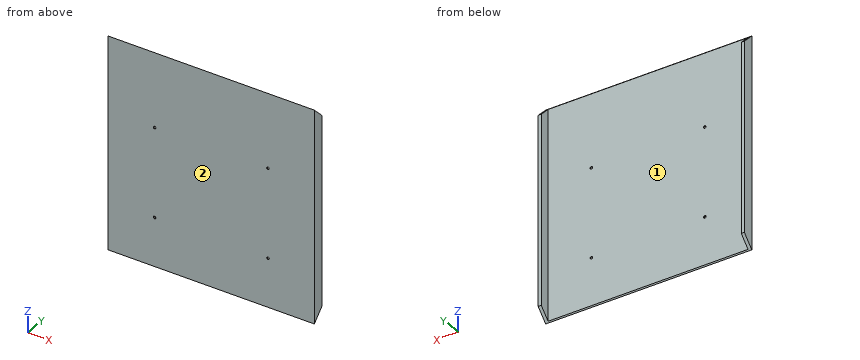
from build123d import *

# Parameters (mm, degrees)
SKETCH1_W           = 200
SKETCH1_H           = 225
SKETCH1_R           = 1.25
BOSS_EXTRUDE1_DEPTH = 1
SKETCH2_W           = 3
SKETCH2_H           = 225
BOSS_EXTRUDE2_DEPTH = 10


with BuildPart() as part:
    # Sketch1 → Boss-Extrude1 (new body)
    with BuildSketch(Plane(origin=(0, 0, 0), x_dir=(1, 0, 0), z_dir=(0, 1, 0))):
        with Locations((100, -112.5)):
            Rectangle(SKETCH1_W, SKETCH1_H)
        with Locations(Location((45, -56.5, 0), (0, 0, 270))):
            Circle(SKETCH1_R, mode=Mode.SUBTRACT)
        with Locations(Location((155, -56.5, 0), (0, 0, 90))):
            Circle(SKETCH1_R, mode=Mode.SUBTRACT)
        with Locations(Location((45, -143.5, 0), (0, 0, 270))):
            Circle(SKETCH1_R, mode=Mode.SUBTRACT)
        with Locations(Location((155, -143.5, 0), (0, 0, 90))):
            Circle(SKETCH1_R, mode=Mode.SUBTRACT)
    extrude(amount=BOSS_EXTRUDE1_DEPTH)

    # Sketch2 → Boss-Extrude2 (add)
    with BuildSketch(Plane(origin=(0, 1, 0), x_dir=(1, 0, 0), z_dir=(0, 1, 0))):
        with Locations((1.5, -112.5)):
            Rectangle(SKETCH2_W, SKETCH2_H)
        with Locations((198.5, -112.5)):
            Rectangle(SKETCH2_W, SKETCH2_H)
    extrude(amount=BOSS_EXTRUDE2_DEPTH)

    # Chamfer7
    # the kernel refuses this chamfer: 20 mm, written as the material it takes off along each edge
    with BuildSketch(Plane(origin=(-123.440783422, 11, 0), x_dir=(0, -0.9996219169112968, -0.027495876610586372), z_dir=(1, 0, 0))) as chamfer7_piece_1:
        with BuildLine():
            Line((20.573463904, 0), (-1.130943098, -20.54235587))
            Line((-1.130943098, -20.54235587), (-1.530791864, -20.53135752))
            ThreePointArc((-1.530791864, -20.53135752), (-0.682584541, -10.267956593), (-0.399848767, 0.010998351))
            Line((-0.399848767, 0.010998351), (0.010998351, 0.399848767))
            ThreePointArc((0.010998351, 0.399848767), (10.289953294, 0.117112992), (20.584462254, 0.399848767))
            Line((20.584462254, 0.399848767), (20.573463904, 0))
        make_face()
    extrude(amount=249.881566845, mode=Mode.SUBTRACT)
    with BuildSketch(Plane(origin=(323.440783422, 11, 0), x_dir=(0, -0.9996219169112968, -0.027495876610586372), z_dir=(-1, 0, 0))) as chamfer7_piece_2:
        with BuildLine():
            Line((20.573463904, 0), (-1.130943098, 20.54235587))
            Line((-1.130943098, 20.54235587), (-1.530791864, 20.53135752))
            ThreePointArc((-1.530791864, 20.53135752), (-0.682584541, 10.267956593), (-0.399848767, -0.010998351))
            Line((-0.399848767, -0.010998351), (0.010998351, -0.399848767))
            ThreePointArc((0.010998351, -0.399848767), (10.289953294, -0.117112992), (20.584462254, -0.399848767))
            Line((20.584462254, -0.399848767), (20.573463904, 0))
        make_face()
    extrude(amount=249.881566845, mode=Mode.SUBTRACT)

    # Chamfer8
    # the kernel refuses this chamfer: 20 mm, written as the material it takes off along each edge
    with BuildSketch(Plane(origin=(126.440783422, 11, 225), x_dir=(0, 0.027495876610586403, -0.9996219169112968), z_dir=(-1, 0, 0))) as chamfer8_piece_1:
        with BuildLine():
            Line((20.573463904, 0), (-1.130943098, 20.54235587))
            Line((-1.130943098, 20.54235587), (-1.530791864, 20.53135752))
            ThreePointArc((-1.530791864, 20.53135752), (-0.682584541, 10.267956593), (-0.399848767, -0.010998351))
            Line((-0.399848767, -0.010998351), (0.010998351, -0.399848767))
            ThreePointArc((0.010998351, -0.399848767), (10.289953294, -0.117112992), (20.584462254, -0.399848767))
            Line((20.584462254, -0.399848767), (20.573463904, 0))
        make_face()
    extrude(amount=249.881566845, mode=Mode.SUBTRACT)
    with BuildSketch(Plane(origin=(73.559216578, 11, 225), x_dir=(0, 0.027495876610586403, -0.9996219169112968), z_dir=(1, 0, 0))) as chamfer8_piece_2:
        with BuildLine():
            Line((20.573463904, 0), (-1.130943098, -20.54235587))
            Line((-1.130943098, -20.54235587), (-1.530791864, -20.53135752))
            ThreePointArc((-1.530791864, -20.53135752), (-0.682584541, -10.267956593), (-0.399848767, 0.010998351))
            Line((-0.399848767, 0.010998351), (0.010998351, 0.399848767))
            ThreePointArc((0.010998351, 0.399848767), (10.289953294, 0.117112992), (20.584462254, 0.399848767))
            Line((20.584462254, 0.399848767), (20.573463904, 0))
        make_face()
    extrude(amount=249.881566845, mode=Mode.SUBTRACT)


solid = part.part
Design review of the part built by this model. Coordinates are the model's own, in mm. Face numbers are marked on the shaded views. Round coordinates to 2 decimals unless told otherwise and drop trailing zeros. Order: outer loops, then holes, each group sorted by start corner. A loop starts at its lowest first (then second) coordinate and runs counter-clockwise, first axis right, second up. Notation, with made-up numbers: M 88.5,60 L 104.5,60 A16 ccw 104.5,75 Z; hole C 38,72 d6. An arc over 180 degrees is marked long. Answer as CSV lines item,"result". Start each with the question number.
1) Add section A-A (y = 8). Give the boundary of the cut face in (x, z).
2) Add section B-B (z = 149). Give the boundary of the cut face in (x, y).
3) For pin 1 Ø3 at (x, z) = (155, 143.5) entering from +Y; pin 2 Ø1.5 at (x, z) = (45, 56.5) entering from +Y, all flat-tipped, find the tip position at first contact; note any pin that passes through.
4) Add section C-C (x = 87). Give the boundary of the cut face in (y, z).
5) Wall thickness on line 1 along X through (y, z) = (0.45, 143.5); line 2 along X through (y, z) = (6, 186.5); line 3 along Y through (x, z) = (75, 104.5): over which ranges is each line inside the solid? List them lowest first. Write a range as [from, to].
6) The part is to be moulded in two halves that separate along X. For the marked faces 1 and 2, say which applies: +X half, -X half, draft (parallel to the pull), parting line (faces both ways), or undercut.
Resolved:
1,outline,"M 0,17 L 3,17 L 3,208 L 0,208 Z; M 197,17 L 200,17 L 200,208 L 197,208 Z"
2,outline,"M 0,0 L 200,0 L 200,11 L 197,11 L 197,1 L 3,1 L 3,11 L 0,11 Z"
3,pin 1,"y = 1"
3,pin 2,"through"
4,outline,"M 0,9 L 1,10 L 1,215 L 0,216 Z"
5,line 1,"[0, 43.75], [46.25, 153.75], [156.25, 200]"
5,line 2,"[0, 3], [197, 200]"
5,line 3,"[0, 1]"
6,face 1,"undercut"
6,face 2,"draft"
